The model under review builds one solid part; all positions refer to its coordinate system, in mm. Face numbers are marked on the shaded views. A direction names the side the tool comes from. Coordinates: 2 decimals unless noted, no trailing zeros. Order: outer loops, then holes, each group sorted by start corner. A loop starts at its lowest first (then second) coordinate and runs counter-clockwise, first axis right, second up.
```python
from build123d import *

# Parameters (mm, degrees)
F0_W      = 79
F0_H      = 78
F1_DEPTH  = 5
F2_W      = 13
F2_H      = 78
F3_DEPTH  = 5
F4_W      = 8.25
F4_H      = 1.4
F5_DEPTH  = 78.001
F6_R      = 1.5
F7_DEPTH  = 30
F8_R      = 3
F9_DEPTH  = 3
F10_W     = 22
F10_H     = 1.4
F11_DEPTH = 25
F12_R     = 1


with BuildPart() as f1:
    # F0 (on Top) → F1 (new body)
    with BuildSketch(Plane.XY):
        with Locations((2.279855, 9.696156)):
            Rectangle(F0_W, F0_H)
    extrude(amount=F1_DEPTH)

    # F2 (on face) → F3 (join)
    with BuildSketch(Plane.XY.offset(5)):
        with Locations((-30.720145, 9.696156)):
            Rectangle(F2_W, F2_H)
        with Locations((35.279855, 9.696156)):
            Rectangle(F2_W, F2_H)
    extrude(amount=F3_DEPTH)

    # F4 (on face) → F5 (cut, through all)
    with BuildSketch(Plane.XZ.offset(29.303844)):
        with Locations((-28.345145, 5.7)):
            Rectangle(F4_W, F4_H)
        with Locations((32.904855, 5.7)):
            Rectangle(F4_W, F4_H)
    extrude(amount=-F5_DEPTH, mode=Mode.SUBTRACT)

    # F6 (on face) → F7 (cut)
    with BuildSketch(Plane.XY.offset(5)):
        with Locations((-17.220145, 38.196156)):
            Circle(F6_R)
        with Locations((21.779855, 38.196156)):
            Circle(F6_R)
        with Locations((-17.220145, -18.803844)):
            Circle(F6_R)
        with Locations((21.779855, -18.803844)):
            Circle(F6_R)
    extrude(amount=-F7_DEPTH, mode=Mode.SUBTRACT)

    # F8 (on face) → F9 (cut)
    with BuildSketch(Plane.XY.offset(5)):
        with Locations((-17.220145, 38.196156)):
            Circle(F8_R)
        with Locations((21.779855, 38.196156)):
            Circle(F8_R)
        with Locations((-17.220145, -18.803844)):
            Circle(F8_R)
        with Locations((21.779855, -18.803844)):
            Circle(F8_R)
    extrude(amount=-F9_DEPTH, mode=Mode.SUBTRACT)

    # F10 (on face) → F11 (cut)
    with BuildSketch(Plane.XZ.offset(29.303844)):
        with Locations((1.356391, 0.7)):
            Rectangle(F10_W, F10_H)
    extrude(amount=-F11_DEPTH, mode=Mode.SUBTRACT)

    # F12
    f12_edges = [f1.edges().sort_by_distance(p)[0] for p in [
        (-24.220145, 9.696156, 10),
        (28.779855, 9.696156, 10),
        (35.279855, -29.303844, 10),
        (-30.720145, -29.303844, 10),
        (-30.720145, 48.696156, 10),
        (35.279855, 48.696156, 10),
        (32.904855, -29.303844, 6.4),
        (-28.345145, -29.303844, 6.4),
        (41.779855, 9.696156, 10),
        (-37.220145, 9.696156, 10),
    ]]
    fillet(f12_edges, radius=F12_R)


solid = f1.part
```
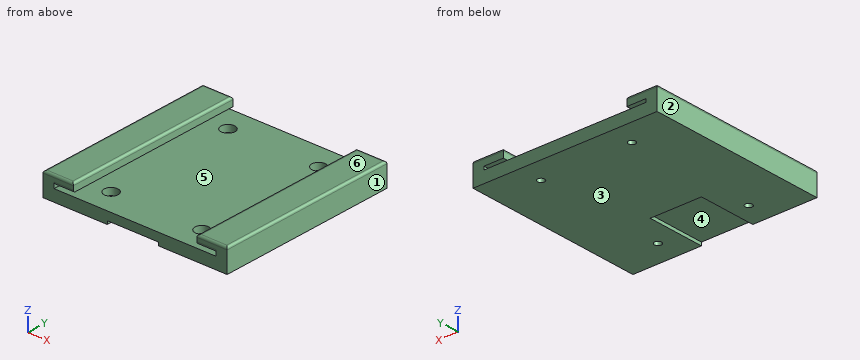
(1) We need section D-D, the plane x = 5. Write out the cut boundary in (y, z).
A:
outline: (-29.3, 1.4) - (-4.3, 1.4) - (-4.3, 0) - (48.7, 0) - (48.7, 5) - (-29.3, 5) - close
(2) We need section B-B, the plane x = 21.5. Write out the cut boundary in (y, z).
A:
outline: (-29.3, 0) - (-20.28, 0) - (-20.28, 2) - (-21.79, 2) - (-21.79, 5) - (-29.3, 5) - close; (-17.33, 0) - (36.72, 0) - (36.72, 2) - (35.21, 2) - (35.21, 5) - (-15.82, 5) - (-15.82, 2) - (-17.33, 2) - close; (39.67, 0) - (48.7, 0) - (48.7, 5) - (41.18, 5) - (41.18, 2) - (39.67, 2) - close
(3) We need section A-A, the plane y = -9.5. Write out the cut boundary in (x, z), and give its area (3 significant figures).
A:
outline: (-37.22, 0) - (-9.64, 0) - (-9.64, 1.4) - (12.36, 1.4) - (12.36, 0) - (41.78, 0) - (41.78, 9) arc R1 ccw to (40.78, 10) - (29.78, 10) arc R1 ccw to (28.78, 9) - (28.78, 6.4) - (37.03, 6.4) - (37.03, 5) - (-32.47, 5) - (-32.47, 6.4) - (-24.22, 6.4) - (-24.22, 9) arc R1 ccw to (-25.22, 10) - (-36.22, 10) arc R1 ccw to (-37.22, 9) - close
area: 470 mm2
(4) For pin 1 Ø6.5 at (x, y) = (-17, 37) entering from +Z; pin 2 Ø3.5 at (x, y) = (21.78, 38.2) entering from +Z; pin 3 Ø11 at (x, y) = (6.5, -22) entering from -Z, all flat-tipped, find the tip position at first contact; note any pin that passes through.
A:
pin 1: stops at z = 5
pin 2: stops at z = 2
pin 3: stops at z = 1.4
(5) Draft analysis for pull direction X (two halves, no side actions). For the marked faces 1, 2, 3 and 4, state which applies: released by +X, released by -X, zero draft, split by the parting line, or undercut.
A:
face 1: released by +X
face 2: released by -X
face 3: zero draft
face 4: undercut
(6) We need section C-C, the plane z = 3. Write out the cut boundary in (x, y), and give its area (3 significant figures).
A:
outline: (-37.22, -29.3) - (41.78, -29.3) - (41.78, 48.7) - (-37.22, 48.7) - close; hole circle Ø6 at (-17.22, -18.8); hole circle Ø6 at (-17.22, 38.2); hole circle Ø6 at (21.78, -18.8); hole circle Ø6 at (21.78, 38.2)
area: 6,050 mm2
(7) Machinability: for the marked faces 5 and 6, which of the approach directions +Z, -Z, +X, -X, +Y, -Y give a long, thin tool a straight path to every point of the face, cutting with its end or side? Answer none if there is none.
A:
face 5: +Y, -Y
face 6: +Z, +X, -X, +Y, -Y
(8) Wall thickness on probe 1 along Z at (x, y) = (35, 37); probe 2 along X at (y, z) = (24, 9); probe 3 along Z at (x, y) = (-6, 44.5): over which ranges is each line inside the solid? List them lowest first.
A:
probe 1: z = 0 to 5, 6.4 to 10
probe 2: x = -37.22 to -24.22, 28.78 to 41.78
probe 3: z = 0 to 5
